The model under review builds one solid part; all positions refer to its coordinate system, in mm. A direction names the side the tool comes from. Coordinates: 2 decimals unless noted, no trailing zeros. Loops run counter-clockwise (first coordinate to the right, second up) from the corner with the lowest first, then second, coordinate; pieces in that order, holes last. Notation, with made-up numbers: M 36,-25.75 L 79,-25.75 A17 cw 79,-7.75 Z; hole C 48,11 d11. An arc over 180 degrees is marked long. One line per item, written item: value.
```python
from build123d import *

# Parameters (mm, degrees)
BOSS_EXTRUDE1_DEPTH = 1.5
SKETCH2_W           = 1.5
SKETCH2_H           = 225
BOSS_EXTRUDE2_DEPTH = 45
CHAMFER1_SIZE       = 2
FILLET1_R           = 1
SKETCH3_R           = 2.25
CUT_EXTRUDE1_DEPTH  = 2.5


with BuildPart() as part:
    # Sketch1 → Boss-Extrude1 (new body)
    with BuildSketch(Plane.XY):
        Polygon((-12.96728972, 188.376168224), (12.03271028, 188.376168224), (12.03271028, -36.623831776), (-7.96728972, -36.623831776), (-7.96728972, -26.623831776), (-12.96728972, -26.623831776), align=None)
    extrude(amount=BOSS_EXTRUDE1_DEPTH)

    # Sketch2 → Boss-Extrude2 (add)
    with BuildSketch(Plane.XY.offset(1.5)):
        with Locations((11.28271028, 75.876168224)):
            Rectangle(SKETCH2_W, SKETCH2_H)
    extrude(amount=BOSS_EXTRUDE2_DEPTH)

    # Chamfer1
    chamfer1_edges = [part.edges().sort_by_distance(p)[0] for p in [
        (-12.96728972, 188.376168224, 0.75),
        (11.28271028, 188.376168224, 46.5),
        (11.28271028, -36.623831776, 46.5),
    ]]
    chamfer(chamfer1_edges, length=CHAMFER1_SIZE)

    # Fillet1
    fillet1_edges = [part.edges().sort_by_distance(p)[0] for p in [
        (12.03271028, 75.876168224, 0),
    ]]
    fillet(fillet1_edges, radius=FILLET1_R)

    # Sketch3 → Cut-Extrude1 (cut, through all)
    with BuildSketch(Plane.XY.offset(1.5)):
        with Locations((3.03271028, 177.946548893)):
            Circle(SKETCH3_R)
        with Locations((3.03271028, -29.014631464)):
            Circle(SKETCH3_R)
    extrude(amount=-CUT_EXTRUDE1_DEPTH, mode=Mode.SUBTRACT)


solid = part.part
```
(1) Add section B-B on z = 41. State the section outline as (x, y) points.
Checks:
outline: M 10.53,-36.62 L 12.03,-36.62 L 12.03,188.38 L 10.53,188.38 Z
(2) Add section A-A on y = 7. State the section outline as (x, z) points.
Checks:
outline: M -12.97,0 L 11.03,0 A1 ccw 12.03,1 L 12.03,46.5 L 10.53,46.5 L 10.53,1.5 L -12.97,1.5 Z
(3) Tool access review of faces 4 (the face through (11, -36.624, 16)), 5 (the face through (-1, 77, 1.5)): name each direction out of +Z, -Z, +X, -X, +Y, -Y from which nothing blocks a thin tool from reaching the whole face with its end or side.
Checks:
face 4: +Z, -Z, +X, -X, -Y
face 5: +Z, -X, +Y, -Y
(4) To check wall thickness, follow L1, parallel to X at y = 104.5, z = 42.5; L2, parallel to Z at x = 9.5, y = 22. State the ranges of each line that lie inside material, in increasing order. Write a range as [from, to].
Checks:
L1: [10.53, 12.03]
L2: [0, 1.5]
(5) Draft analysis for pull direction Y (two halves, no side actions). For faces 1 (the face through (11, 188.376, 16)), 2 (the face through (2.54, 175.75, 0.76)), 3 (the face through (10.533, 74, 24)), state which applies: pulls with the +Y half, pulls with the -Y half, needs draft (parallel to the pull), parting line crosses it, or undercut.
Checks:
face 1: pulls with the +Y half
face 2: undercut
face 3: needs draft
(6) Insertion check: pin 1 Ø6 at (y, z) = (79, 41.5) entering from -X; pin 2 Ø6 at (x, y) = (-2, 96.5) entering from -Z; pin 3 Ø8 at (x, z) = (4, 7.5) entering from +Y; pin 4 Ø10 at (x, y) = (3, 133.5) entering from +Z. Each pin has a flat end and moves straight along its axis. Give the tip position at first contact, or say it passes through.
Checks:
pin 1: x = 10.53
pin 2: z = 0
pin 3: through
pin 4: z = 1.5
(7) Add section C-C on x = 8.25. State the section outline as (y, z) points, then the cut area to 4 significant figures.
Checks:
outline: M -36.62,0 L 188.38,0 L 188.38,1.5 L -36.62,1.5 Z
area: 337.5 mm^2
